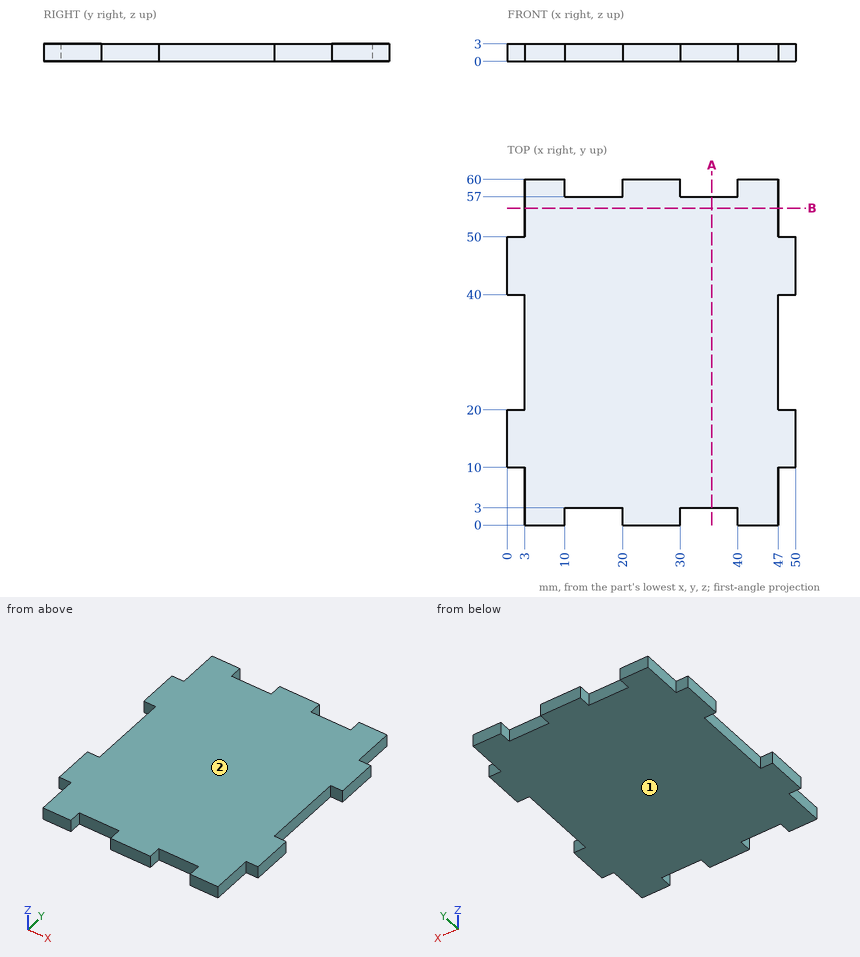
Geometry check sheet. Reference: drawing and pictorial views, mm from the part's lowest x, y, z. Round coordinates to 2 decimals unless told otherwise and drop trailing zeros. Order: outer loops, then holes, each group sorted by start corner. A loop starts at its lowest first (then second) coordinate and runs counter-clockwise, first axis right, second up. Notation, with made-up numbers: M 53.5,5 L 57.5,5 A18 cw 57.5,37 Z; hole C -3,76.25 d10. An arc over 180 degrees is marked long. Write item = value, one per line.
Q1. Scan lines: line 1 (X direction, y = 22, z = 1.6); line 2 (Y direction, x = 19, z = 1.6). Record each from-to range of solid material in increasing order.
Answer block:
line_1 = 3 to 47
line_2 = 3 to 57
Q2. Depth check by flat-ended pin: pin 1 Ø1.5 at (y, z) = (2, 1.5) entering from +X; pin 2 Ø0.9 at (x, z) = (48, 2) entering from +Y; pin 3 Ø1.5 at (y, z) = (59, 1.5) entering from -X. Enter the tip coordinate at first touch or a pass-through.
Answer block:
pin_1 = 47
pin_2 = 50
pin_3 = 3
Q3. Section check B-B (y = 55). Enter the section's corners in (x, z), plus the area to 3 significant figures.
Answer block:
outline = M 3,0 L 47,0 L 47,3 L 3,3 Z
area = 132 mm^2
Q4. Section check A-A (x = 35.5). Enter the section's corners in (y, z), plus the area to 3 significant figures.
Answer block:
outline = M 3,0 L 57,0 L 57,3 L 3,3 Z
area = 162 mm^2
Q5. Release check for a two-part mould opening along Z. For the marked faces 1 and 2 record: released by +Z, released by -Z, zero draft, split by the parting line, or undercut.
Answer block:
face_1 = released by -Z
face_2 = released by +Z
